from build123d import *

# Parameters (mm, degrees)
SKETCH_2_R          = 1.5
CUT_EXTRUDE_1_DEPTH = 10


with BuildPart() as part:
    # 草图1 → 旋转1 (revolve)
    with BuildSketch(Plane.XY, mode=Mode.PRIVATE) as revolve_1_sk:
        Polygon((-2.579365079, 1.5), (-2.579365079, 10), (-0.079365079, 10), (-0.079365079, 4.5), (1.920634921, 4.5), (1.920634921, 2.95), (-1.989795918, 2.95), (-1.989795918, 1.5), align=None)
    revolve(revolve_1_sk.sketch.rotate(Axis((-8.588435374, 0, 0), (1, 0, 0)), 90), axis=Axis((-8.588435374, 0, 0), (1, 0, 0)))

    # 草图2 → 切除-拉伸1 (cut)
    with BuildSketch(Plane(origin=(-0.079365079, 0, 0), x_dir=(0, 0, -1), z_dir=(1, 0, 0))):
        with Locations((0, 7)):
            Circle(SKETCH_2_R)
        with Locations((7, 0)):
            Circle(SKETCH_2_R)
        with Locations((0, -7)):
            Circle(SKETCH_2_R)
        with Locations((-7, 0)):
            Circle(SKETCH_2_R)
    extrude(amount=-CUT_EXTRUDE_1_DEPTH, mode=Mode.SUBTRACT)


solid = part.part
Here's how the part is built. I have some questions about the finished solid (model axes, mm). A direction names the side the tool comes from. Give positions to 0.01 mm unless a question says otherwise; leave off trailing zeros. Order: outer loops, then holes, each group sorted by start corner. A loop starts at its lowest first (then second) coordinate and runs counter-clockwise, first axis right, second up. Notation, with made-up numbers: M 89,-35 L 96,-35 A35 cw 96,0 Z; hole C -31.75,-27 d2. An arc over 180 degrees is marked long. Answer as a JSON object with one key per item and string values. Group by question number.
1) Please list where these lines run through material, in increasing order: L1, parallel to Y at x = -1.9, z = 0; L2, parallel to Y at x = -2.35, z = 0; L3, parallel to Y at x = 0.35, z = 0. Write a range as [from, to].
2) I'm going to push flat-ended pins straight in: pin 1 Ø1.8 at (y, z) = (0, 0) entering from -X; pin 2 Ø3.5 at (y, z) = (0, 0) entering from +X; pin 3 Ø4 at (y, z) = (-3.5, -6.5) entering from +X; pin 4 Ø1.5 at (x, y) = (-0.5, -4) entering from -Z. Where does each tip first touch, or does it pass through?
3) Suppose I cut it at B-B, the plane x = -2.3. Write out the boundary of the cut face in (y, z).
4) Suppose I cut it at D-D, the plane z = -5.75. Write out the boundary of the cut face in (x, y), plus the area to 3 significant figures.
5) On a 3-axis mill with a long thin cutter (end or side, diameter ignored), from which of +Z, -Z, +X, -X, +Y, -Y can I reach the whole of each face in a straight line? I mean faces 4 (the cylindrical face through (-2.29, -0.45, 1.43)), 5 (the cylindrical face through (-0.062, -0.13, -2.947)). Say none if no direction works.
6) We'd pull the mould along Z, two halves only. Please class faces 1 (the flat face through (-0.079, 2.1, 4.3)), 2 (the cylindrical face through (-1.31, 0.07, -5.5)), 3 (the cylindrical face through (0.93, -3.04, -3.32)): pulls with the +Z half, pulls with the -Z half, needs draft (parallel to the pull), parting line crosses it, or undercut.
7) Suppose I cut it at A-A, the plane y = 0. Write out the boundary of the cut face in (x, z).
8) Suppose I cut it at C-C, the plane y = -7. Write out the boundary of the cut face in (x, z).
Results found:
{
 "1": {"L1": "[-10, -8.5], [-5.5, -2.95], [2.95, 5.5], [8.5, 10]", "L2": "[-10, -8.5], [-5.5, -1.5], [1.5, 5.5], [8.5, 10]", "L3": "[-4.5, -2.95], [2.95, 4.5]"},
 "2": {"pin 1": "through", "pin 2": "x = -1.99", "pin 3": "x = -0.08", "pin 4": "z = -9.46"},
 "3": {"outline": "C 0,0 d20; hole C -7,0 d3; hole C 0,-7 d3; hole C 0,0 d3; hole C 0,7 d3; hole C 7,0 d3"},
 "4": {"outline": "M -2.58,-8.18 L -0.08,-8.18 L -0.08,-0.83 L -2.58,-0.83 Z; M -2.58,0.83 L -0.08,0.83 L -0.08,8.18 L -2.58,8.18 Z", "area": "36.8 mm²"},
 "5": {"face 4": "+X, -X", "face 5": "+X"},
 "6": {"face 1": "needs draft", "face 2": "undercut", "face 3": "parting line crosses it"},
 "7": {"outline": "M -2.58,-10 L -0.08,-10 L -0.08,-8.5 L -2.58,-8.5 Z; M -2.58,-5.5 L -0.08,-5.5 L -0.08,-4.5 L 1.92,-4.5 L 1.92,-2.95 L -1.99,-2.95 L -1.99,-1.5 L -2.58,-1.5 Z; M -2.58,1.5 L -1.99,1.5 L -1.99,2.95 L 1.92,2.95 L 1.92,4.5 L -0.08,4.5 L -0.08,5.5 L -2.58,5.5 Z; M -2.58,8.5 L -0.08,8.5 L -0.08,10 L -2.58,10 Z"},
 "8": {"outline": "M -2.58,-7.14 L -0.08,-7.14 L -0.08,-1.5 L -2.58,-1.5 Z; M -2.58,1.5 L -0.08,1.5 L -0.08,7.14 L -2.58,7.14 Z"}
}
